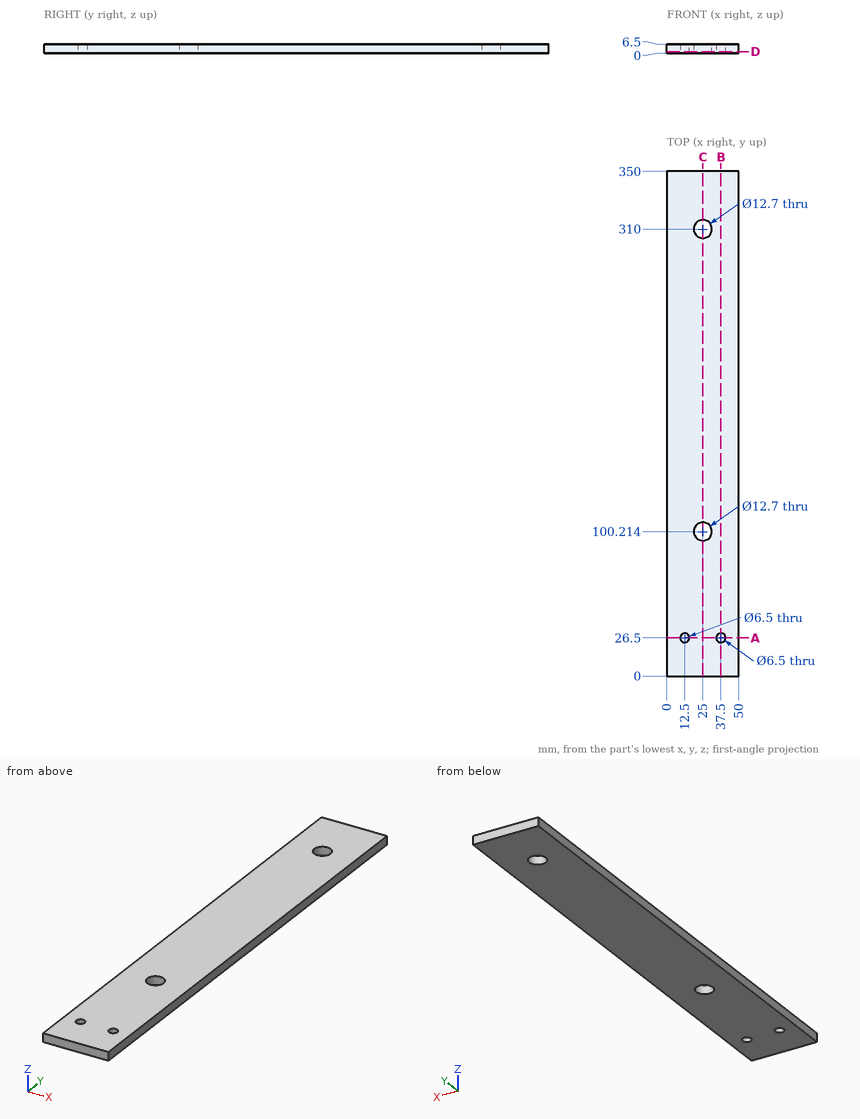
Check sheet for the drawn part. Datum: minimum x, y, z corner. Units: mm. Coordinates: 2 decimals unless noted, no trailing zeros. Loops run counter-clockwise (first coordinate to the right, second up) from the corner with the lowest first, then second, coordinate; pieces in that order, holes last. Notation, with made-up numbers: (-3.5, 14) -> (8.5, 14) arc R25 ccw to (8.5, 32) -> close; hole circle Ø8 at (23.25, 19). An arc over 180 degrees is marked (long way). Answer as CSV lines item,"result".
1) Cross-section at D-D, the plane z = 1.25. Record the cut outline in (x, y), then the cut area to 3 significant figures.
Found:
outline,"(0, 0) -> (50, 0) -> (50, 350) -> (0, 350) -> close; hole circle Ø6.5 at (12.5, 26.5); hole circle Ø12.7 at (25, 100.21); hole circle Ø12.7 at (25, 310); hole circle Ø6.5 at (37.5, 26.5)"
area,"17,200 mm2"
2) Cross-section at C-C, the plane x = 25. Record the cut outline in (y, z), then the cut area to 3 significant figures.
Found:
outline,"(0, 0) -> (93.86, 0) -> (93.86, 6.5) -> (0, 6.5) -> close; (106.56, 0) -> (303.65, 0) -> (303.65, 6.5) -> (106.56, 6.5) -> close; (316.35, 0) -> (350, 0) -> (350, 6.5) -> (316.35, 6.5) -> close"
area,"2,110 mm2"
3) Thickness scan on L1, parallel to Y at x = 37.5, z = 4.75; L2, parallel to Y at x = 25, z = 3; L3, parallel to X at y = 29, z = 5. Record the ranges inside material, lowest first. Write a range as from..to.
Found:
L1,"y = 0..23.25, 29.75..350"
L2,"y = 0..93.86, 106.56..303.65, 316.35..350"
L3,"x = 0..10.42, 14.58..35.42, 39.58..50"
4) Cross-section at B-B, the plane x = 37.5. Record the cut outline in (y, z), then the cut area to 3 significant figures.
Found:
outline,"(0, 0) -> (23.25, 0) -> (23.25, 6.5) -> (0, 6.5) -> close; (29.75, 0) -> (350, 0) -> (350, 6.5) -> (29.75, 6.5) -> close"
area,"2,230 mm2"
5) Cross-section at A-A, the plane y = 26.5. Record the cut outline in (x, z).
Found:
outline,"(0, 0) -> (9.25, 0) -> (9.25, 6.5) -> (0, 6.5) -> close; (15.75, 0) -> (34.25, 0) -> (34.25, 6.5) -> (15.75, 6.5) -> close; (40.75, 0) -> (50, 0) -> (50, 6.5) -> (40.75, 6.5) -> close"
